Part model, mm, in its own coordinate system. A direction names the side the tool comes from. Coordinates: 2 decimals unless noted, no trailing zeros. Write each loop counter-clockwise with the first axis right and the second up, starting at its lowest first coordinate (ties: lowest second). Pieces come first, ordered by that corner, then holes. Notation, with made-up numbers: M 15.25,64 L 69.25,64 A17 ccw 69.25,94 Z; hole C 72.25,60.5 d7. An arc over 180 degrees is marked long. Use a Markdown table: item, result. Add a question column.
Q1. Tool access for faces 1 (the flat face through (-1415, -915, 30)), 2 (the flat face through (-1014, 0, 114)), 3 (the flat face through (-213.452, -493, 226)): list every direction of +Z, -Z, +X, -X, +Y, -Y with a clear straight run to the whole face (end or side of a thin tool).
Q2. Mould opens along X. For faces 4 (the flat face through (-2000, -493, 197)), 5 (the flat face through (-1024, -493, 316.173)), 6 (the flat face through (-1014, -493, 400)) say: released by +X, released by -X, zero draft, split by the parting line, or undercut.
Q3. Wall check: L1, parallel to Y at x = -585, z = 6; L2, parallel to X at y = -561, z = 259.5; L3, parallel to Z at x = -700, y = -322. Give the ranges that are in metal, low to high. Write a range as from..to.
Q4. Slice it at A-A on x = -1299.5. Write the cut outline in (y, z).
Q5. Slice it at C-C on z = 198. Write the cut outline in (x, y).
Q6. Slice it at D-D on x = -585. Write the cut outline in (y, z), then the cut area to 3 significant figures.
Q7. Slice it at B-B on y = -500. Write the cut outline in (x, z), then the cut area to 3 significant figures.
from build123d import *

# Parameters (mm, degrees)
F0_W      = 2000
F0_H      = 425
F0_W_2    = 1598.034471
F0_H_2    = 178.189233
F1_DEPTH  = 1000
F1_FACE_W = 2000
F1_FACE_H = 1000
F2_DEPTH  = 25
F3_R      = 35
F4_DEPTH  = 30
F5_R      = 225
F6_DEPTH  = 122


with BuildPart() as f1:
    # F0 (on Front) → F1 (new body)
    with BuildSketch(Plane.XZ):
        with Locations((-1000, 212.5)):
            Rectangle(F0_W, F0_H)
        with Locations((-1012.46877, 227.07834)):
            Rectangle(F0_W_2, F0_H_2, mode=Mode.SUBTRACT)
    extrude(amount=F1_DEPTH)

    # F1_face (on face) → F2 (cut)
    with BuildSketch(Plane(origin=(-1000, -500, 425), x_dir=(1, 0, 0), z_dir=(0, 0, 1))):
        Rectangle(F1_FACE_W, F1_FACE_H)
    extrude(amount=-F2_DEPTH, mode=Mode.SUBTRACT)

    # F3 (on Top) → F4 (cut)
    with BuildSketch(Plane.XY):
        with Locations((-1415, -85)):
            Circle(F3_R)
        with Locations((-1415, -915)):
            Circle(F3_R)
        with Locations((-585, -915)):
            Circle(F3_R)
        with Locations((-585, -90)):
            Circle(F3_R)
    extrude(amount=F4_DEPTH, mode=Mode.SUBTRACT)

    # F5 (on face) → F6 (cut)
    with BuildSketch(Plane(origin=(0, 0, 0), x_dir=(1, 0, 0), z_dir=(0, 0, -1))):
        with Locations((-1000, 500)):
            Circle(F5_R)
    extrude(amount=-F6_DEPTH, mode=Mode.SUBTRACT)


solid = f1.part
Recorded:
| question | item | result |
|---|---|---|
| 1 | face 1 | -Z |
| 1 | face 2 | +Z, -Z, +X, -X, +Y |
| 1 | face 3 | +Y, -Y |
| 2 | face 4 | released by -X |
| 2 | face 5 | undercut |
| 2 | face 6 | zero draft |
| 3 | L1 | -1000..-950, -880..-125, -55..0 |
| 3 | L2 | -2000..-1811.49, -213.45..0 |
| 3 | L3 | 0..137.98, 316.17..400 |
| 4 | outline | M -1000,0 L 0,0 L 0,137.98 L -1000,137.98 Z; M -1000,316.17 L 0,316.17 L 0,400 L -1000,400 Z |
| 5 | outline | M -2000,-1000 L -1811.49,-1000 L -1811.49,0 L -2000,0 Z; M -213.45,-1000 L 0,-1000 L 0,0 L -213.45,0 Z |
| 6 | outline | M -1000,0 L -950,0 L -950,30 L -880,30 L -880,0 L -125,0 L -125,30 L -55,30 L -55,0 L 0,0 L 0,137.98 L -1000,137.98 Z; M -1000,316.17 L 0,316.17 L 0,400 L -1000,400 Z |
| 6 | area | 218,000 mm² |
| 7 | outline | M -2000,0 L -1225,0 L -1225,122 L -775,122 L -775,0 L 0,0 L 0,400 L -2000,400 Z; hole M -1811.49,137.98 L -213.45,137.98 L -213.45,316.17 L -1811.49,316.17 Z |
| 7 | area | 460,000 mm² |
